For this review, take the finished solid that the model builds, in its own axes (mm). A direction names the side the tool comes from. Give positions to 0.01 mm unless a question says otherwise; leave off trailing zeros. Loops run counter-clockwise (first coordinate to the right, second up) from the corner with the lowest first, then second, coordinate; pieces in that order, holes last.
```python
from build123d import *

# Parameters (mm, degrees)
SKETCH_1_R      = 1.6
SKETCH_1_R_2    = 2.6
EXTRUDE_1_DEPTH = 1.5


with BuildPart() as part:
    # 草图1 → 凸台-拉伸1 (new, symmetric)
    with BuildSketch(Plane.XY):
        with BuildLine():
            Line((60, 77.5), (-30, 77.5))
            ThreePointArc((-30, 77.5), (-37.071067812, 74.571067812), (-40, 67.5))
            Line((-40, 67.5), (-40, 29.5))
            ThreePointArc((-40, 29.5), (-39.238795325, 25.673165676), (-37.071067812, 22.428932188))
            Line((-37.071067812, 22.428932188), (-17.928932188, 3.286796564))
            ThreePointArc((-17.928932188, 3.286796564), (-15.761204675, 0.042563076), (-15, -3.784271247))
            Line((-15, -3.784271247), (-15, -12.5))
            ThreePointArc((-15, -12.5), (-17.928932188, -19.571067812), (-25, -22.5))
            Line((-25, -22.5), (-30, -22.5))
            ThreePointArc((-30, -22.5), (-37.071067812, -25.428932188), (-40, -32.5))
            Line((-40, -32.5), (-40, -50))
            ThreePointArc((-40, -50), (-38.535533906, -53.535533906), (-35, -55))
            Line((-35, -55), (60, -55))
            ThreePointArc((60, -55), (63.535533906, -53.535533906), (65, -50))
            Line((65, -50), (65, -32.5))
            ThreePointArc((65, -32.5), (62.071067812, -25.428932188), (55, -22.5))
            Line((55, -22.5), (50, -22.5))
            ThreePointArc((50, -22.5), (42.928932188, -19.571067812), (40, -12.5))
            Line((40, -12.5), (40, 47.5))
            ThreePointArc((40, 47.5), (42.928932188, 54.571067812), (50, 57.5))
            Line((50, 57.5), (60, 57.5))
            ThreePointArc((60, 57.5), (63.535533906, 58.964466094), (65, 62.5))
            Line((65, 62.5), (65, 72.5))
            ThreePointArc((65, 72.5), (63.535533906, 76.035533906), (60, 77.5))
        make_face()
        with Locations((-30, 67.5)):
            Circle(SKETCH_1_R, mode=Mode.SUBTRACT)
        with Locations((-10, 67.5)):
            Circle(SKETCH_1_R, mode=Mode.SUBTRACT)
        with Locations((-10, -32.5)):
            Circle(SKETCH_1_R, mode=Mode.SUBTRACT)
        with Locations((-30, -32.5)):
            Circle(SKETCH_1_R, mode=Mode.SUBTRACT)
        with Locations((10, 10)):
            Circle(SKETCH_1_R_2, mode=Mode.SUBTRACT)
        with Locations((15, 67.5)):
            Circle(SKETCH_1_R, mode=Mode.SUBTRACT)
        with Locations((55, 67.5)):
            Circle(SKETCH_1_R, mode=Mode.SUBTRACT)
        with Locations((32, 10)):
            Circle(SKETCH_1_R, mode=Mode.SUBTRACT)
        with Locations((35, 67.5)):
            Circle(SKETCH_1_R, mode=Mode.SUBTRACT)
        with Locations((40, -32.5)):
            Circle(SKETCH_1_R, mode=Mode.SUBTRACT)
        with Locations((55, -32.5)):
            Circle(SKETCH_1_R, mode=Mode.SUBTRACT)
        with Locations((-10, -12.5)):
            Circle(SKETCH_1_R, mode=Mode.SUBTRACT)
        with Locations((-10, 7.5)):
            Circle(SKETCH_1_R, mode=Mode.SUBTRACT)
        with Locations((-10, 47.5)):
            Circle(SKETCH_1_R, mode=Mode.SUBTRACT)
        with Locations((-30, 47.5)):
            Circle(SKETCH_1_R, mode=Mode.SUBTRACT)
        with BuildLine():
            Line((-32, 29.5), (-28, 29.5))
            ThreePointArc((-28, 29.5), (-26.25, 27.75), (-28, 26))
            Line((-28, 26), (-32, 26))
            ThreePointArc((-32, 26), (-33.75, 27.75), (-32, 29.5))
        make_face(mode=Mode.SUBTRACT)
        with BuildLine():
            Line((-12, 29.5), (-8, 29.5))
            ThreePointArc((-8, 29.5), (-6.25, 27.75), (-8, 26))
            Line((-8, 26), (-12, 26))
            ThreePointArc((-12, 26), (-13.75, 27.75), (-12, 29.5))
        make_face(mode=Mode.SUBTRACT)
        with BuildLine():
            Line((-12, 61), (-8, 61))
            ThreePointArc((-8, 61), (-6.25, 59.25), (-8, 57.5))
            Line((-8, 57.5), (-12, 57.5))
            ThreePointArc((-12, 57.5), (-13.75, 59.25), (-12, 61))
        make_face(mode=Mode.SUBTRACT)
        with BuildLine():
            Line((-32, 61), (-28, 61))
            ThreePointArc((-28, 61), (-26.25, 59.25), (-28, 57.5))
            Line((-28, 57.5), (-32, 57.5))
            ThreePointArc((-32, 57.5), (-33.75, 59.25), (-32, 61))
        make_face(mode=Mode.SUBTRACT)
        with BuildLine():
            Line((6, -7), (6, -31))
            ThreePointArc((6, -31), (7.171572875, -33.828427125), (10, -35))
            Line((10, -35), (26, -35))
            ThreePointArc((26, -35), (28.828427125, -33.828427125), (30, -31))
            Line((30, -31), (30, -7))
            ThreePointArc((30, -7), (28.828427125, -4.171572875), (26, -3))
            Line((26, -3), (10, -3))
            ThreePointArc((10, -3), (7.171572875, -4.171572875), (6, -7))
        make_face(mode=Mode.SUBTRACT)
        with BuildLine():
            Line((10, 57.5), (26, 57.5))
            ThreePointArc((26, 57.5), (28.828427125, 56.328427125), (30, 53.5))
            Line((30, 53.5), (30, 29.5))
            ThreePointArc((30, 29.5), (28.828427125, 26.671572875), (26, 25.5))
            Line((26, 25.5), (10, 25.5))
            ThreePointArc((10, 25.5), (7.171572875, 26.671572875), (6, 29.5))
            Line((6, 29.5), (6, 53.5))
            ThreePointArc((6, 53.5), (7.171572875, 56.328427125), (10, 57.5))
        make_face(mode=Mode.SUBTRACT)
    extrude(amount=EXTRUDE_1_DEPTH, both=True)


solid = part.part
```
Q1. Consider section A-A on x = 52. Give the boundary of the cut face in (y, z), plus the area to 4 significant figures.
Answers:
outline: (-55, -1.5) - (-22.5, -1.5) - (-22.5, 1.5) - (-55, 1.5) - close; (57.5, -1.5) - (77.5, -1.5) - (77.5, 1.5) - (57.5, 1.5) - close
area: 157.5 mm2
Q2. Consider section C-C on z = -0.15. Count the separate pieces of the cut face and the enclosed holes in it, plus the area to 3 significant figures.
Answers:
separate pieces: 1
enclosed holes: 21
area: 9,270 mm2
Q3. For pin 1 Ø1 at (x, y) = (8, -8) entering from -Z; pin 2 Ø1 at (y, z) = (-19.5, -1) entering from +X, all flat-tipped, find the tip position at first contact; note any pin that passes through.
Answers:
pin 1: passes through
pin 2: stops at x = 43.39
Q4. Machinability: for faces 1 (the flat face through (-27, -22.5, 0)), 2 (the cylindrical face through (43.01, -19.65, 0.02)), 3 (the flat face through (-30, 57.5, 0)), which of the approach directions +Z, -Z, +X, -X, +Y, -Y give a long, thin tool a straight path to every point of the face, cutting with its end or side? Answer none if there is none.
Answers:
face 1: +Z, -Z, -X
face 2: +Z, -Z, +X
face 3: +Z, -Z
Q5. For probe 1 along X at (y, z) = (67.5, 0); probe 2 along Y at (x, z) = (55, 0.7); probe 3 along Y at (x, z) = (19.5, 0.3), list the stretches that pass through material, from the lowest coordinate up.
Answers:
probe 1: x = -40 to -31.6, -28.4 to -11.6, -8.4 to 13.4, 16.6 to 33.4, 36.6 to 53.4, 56.6 to 65
probe 2: y = -55 to -34.1, -30.9 to -22.5, 57.5 to 65.9, 69.1 to 77.5
probe 3: y = -55 to -35, -3 to 25.5, 57.5 to 77.5
Q6. Mouldability with a two-part tool opening along X and no side actions: class faces 4 (the flat face through (-15, -8, 0)), 5 (the cylindrical face through (28.797, 56.359, 0.021)), 6 (the flat face through (0, 12, 1.5)), 7 (the flat face through (65, -41, 0)) as +X half, -X half, draft (parallel to the pull), parting line (faces both ways), or undercut.
Answers:
face 4: -X half
face 5: undercut
face 6: draft
face 7: +X half
Q7. Consider section B-B on y = 39. Give the boundary of the cut face in (x, z), plus the area to 3 significant figures.
Answers:
outline: (-40, -1.5) - (6, -1.5) - (6, 1.5) - (-40, 1.5) - close; (30, -1.5) - (40, -1.5) - (40, 1.5) - (30, 1.5) - close
area: 168 mm2
